```python
from build123d import *

# Parameters (mm, degrees)
F1_DEPTH = 6.35
F2_R     = 6.3499
F0_R     = 5.08
F3_DEPTH = 6.35
F0_R_2   = 4.826
F4_DEPTH = 6.35
F5_DEPTH = 6.35


# Not quite as in the source:
# - a fillet or chamfer is up to 0.001 mm smaller than in the source, because OpenCascade refuses the exact size


with BuildPart() as f1:
    # F0 (on Front) → F1 (new body, symmetric)
    with BuildSketch(Plane.XZ):
        with BuildLine():
            Line((19.05, 6.35), (-19.05, 6.35))
            ThreePointArc((-19.05, 6.35), (-17.3945407024, 3.3649028089), (-16.821147458, 0))
            ThreePointArc((-16.821147458, 0), (-17.3945407024, -3.3649028089), (-19.05, -6.35))
            Line((-19.05, -6.35), (19.05, -6.35))
            ThreePointArc((19.05, -6.35), (16.821147458, 0), (19.05, 6.35))
        make_face()
    extrude(amount=F1_DEPTH, both=True)

    # F2 (radius 6.35 in the source; OpenCascade refuses exactly that, so slightly less here)
    f2_edges = [f1.edges().sort_by_distance(p)[0] for p in [
        (0, -6.35, 6.35),
        (0, 6.35, 6.35),
        (0, -6.35, -6.35),
        (0, 6.35, -6.35),
    ]]
    fillet(f2_edges, radius=F2_R)

    # F0 (on Front) → F3 (join)
    with BuildSketch(Plane.XZ):
        with BuildLine():
            ThreePointArc((37.141147458, 0), (30.3460502669, 9.5866067556), (19.05, 6.35))
            Line((19.05, 6.35), (19.05, -6.35))
            ThreePointArc((19.05, -6.35), (30.3460502669, -9.5866067556), (37.141147458, 0))
        make_face()
        with Locations((26.981147458, 0)):
            Circle(F0_R, mode=Mode.SUBTRACT)
        with BuildLine():
            Line((19.05, -6.35), (19.05, 6.35))
            ThreePointArc((19.05, 6.35), (16.821147458, 0), (19.05, -6.35))
        make_face()
    extrude(amount=F3_DEPTH)

    # F0 (on Front) → F4 (join)
    with BuildSketch(Plane.XZ):
        with BuildLine():
            Line((-19.05, -6.35), (-19.05, 6.35))
            ThreePointArc((-19.05, 6.35), (-37.141147458, 0), (-19.05, -6.35))
        make_face()
        with Locations((-26.981147458, 0)):
            Circle(F0_R_2, mode=Mode.SUBTRACT)
        with BuildLine():
            ThreePointArc((-16.821147458, 0), (-17.3945407024, 3.3649028089), (-19.05, 6.35))
            Line((-19.05, 6.35), (-19.05, -6.35))
            ThreePointArc((-19.05, -6.35), (-17.3945407024, -3.3649028089), (-16.821147458, 0))
        make_face()
    extrude(amount=-F4_DEPTH)

    # F0 (on Front) → F5 (join, symmetric)
    with BuildSketch(Plane.XZ):
        with Locations((-26.981147458, 0)):
            Circle(F0_R_2)
    extrude(amount=F5_DEPTH, both=True)


solid = f1.part
```
Geometry check sheet. Reference: the model listing, model coordinates, mm. A direction names the side the tool comes from. Coordinates: 2 decimals unless noted, no trailing zeros. Write each loop counter-clockwise with the first axis right and the second up, starting at its lowest first coordinate (ties: lowest second). Pieces come first, ordered by that corner, then holes. Notation, with made-up numbers: M 32,-4 L 62,-4 A25 ccw 62,13 Z; hole C 47,85 d4. An arc over 180 degrees is marked long. One line per item, written item: value. Start each with the question number.
(1) Scan lines: line 1 along X through (y, z) = (-5, -2.5); line 2 along X through (y, z) = (-3.25, -0.5); line 3 along Y through (x, z) = (20, -2.5). Record each from-to range of solid material in increasing order. Write a range as [from, to].
(2) Tool access check on faces 4 (the face through (0.27, -4.44, -4.54)), 5 (the face through (-22.38, -3.22, 1.45)), 6 (the face through (0.27, 4.44, -4.54)), 7 (the face through (-0.27, -4.44, 4.54)). Record the directions out of +Z, -Z, +X, -X, +Y, -Y that give a thin tool (end or side, any length) a straight path to the whole face; none if there is none.
(3) Sectioned sample at C-C, the plane z = 2.75. Enter the section's corners in (x, y).
(4) Depth check by flat-ended pin: pin 1 (11.5 mm diameter, centred on x = 26.98, z = 0, fed in from +Y); pin 2 (6 mm diameter, centred on x = 7.5, y = -2, fed in from +Z); pin 3 (5 mm diameter, centred on x = 13.5, y = 1, fed in from -Z). Enter the tip coordinate at first touch or a pass-through.
(5) Sectioned sample at D-D, the plane x = 26.5. Enter the section's corners in (y, z).
(6) Release check for a two-part mould opening along X. For faces 1 (the face through (16.82, 2.42, -0.1)), 2 (the face through (-16.82, -2.51, 0.1)), 3 (the face through (-26, 6.35, 0)) record: released by +X, released by -X, zero draft, split by the parting line, or undercut.
(7) Sectioned sample at A-A, the plane y = -5.5. Enter the section's corners in (x, z).
Filled sheet:
1. line 1: [-31.11, -22.85], [-17.13, 22.56], [31.4, 36.83]
1. line 2: [-31.78, -22.18], [-16.83, 21.93], [32.04, 37.13]
1. line 3: [-6.35, 0]
2. face 4: -Z, -Y
2. face 5: -Y
2. face 6: -Z, +X, +Y
2. face 7: +Z, -Y
3. outline: M -36.76,0 L -30.95,0 L -30.95,-6.35 L -23.02,-6.35 L -23.02,0 L -17.2,0 L -17.2,-5.72 L 17.2,-5.72 L 17.2,-6.35 L 22.71,-6.35 L 22.71,0 L 17.2,0 L 17.2,5.72 L -17.2,5.72 L -17.2,6.35 L -36.76,6.35 Z; M 31.25,-6.35 L 36.76,-6.35 L 36.76,0 L 31.25,0 Z
4. pin 1: y = 0
4. pin 2: z = 6.35
4. pin 3: z = -6.35
5. outline: M -6.35,-10.15 L 0,-10.15 L 0,-5.06 L -6.35,-5.06 Z; M -6.35,5.06 L 0,5.06 L 0,10.15 L -6.35,10.15 Z
6. face 1: released by +X
6. face 2: undercut
6. face 3: zero draft
7. outline: C -26.98,0 d9.65; M -17.33,-3.17 L 17.33,-3.17 A10.16 ccw long 17.33,3.17 L -17.33,3.17 A10.16 cw Z; hole C 26.98,0 d10.16
